Could you check a few things on this model? Use its own coordinates, in mm. A direction names the side the tool comes from. Coordinates: 2 decimals unless noted, no trailing zeros. Loops run counter-clockwise (first coordinate to the right, second up) from the corner with the lowest first, then second, coordinate; pieces in that order, holes last.
1) Imagine slicing it at A-A on x = 14.5. Please give me the cut outline in (y, z).
2) If I drill on line 1 along X through (y, z) = (-6.25, -3.5); line 2 along X through (y, z) = (-6, -5); line 3 along Z through (x, y) = (10.5, -3), over which ranges is the centre line in solid material (lowest first)?
3) For faces 1 (the face through (-6.226, 4.168, 7.179)), 2 (the face through (11.87, -1.08, 4.88)), which set-ups out of +Z, -Z, +X, -X, +Y, -Y let a thin tool reach every point of the face, with its end or its side?
4) Will these pins go through, and if not, where does the flat tip stop? P1, Ø10, axis at x = 13.5, y = 6.5, coming from the +Z side; P2, Ø1.5, axis at y = 5.5, z = -1.5, coming from the +X side; P3, Ø1, axis at x = 4, y = -3, coming from the +Z side.
Autodesk Inventor part; units mm, degrees
ref_plane "Work Plane1" through (1.525, 0, 0) normal (0, 0, 1) x (1, 0, 0)
ref_plane "YZ Plane" through (0, 0, 0) normal (1, 0, 0) x (0, 1, 0)
ref_plane "XZ Plane" through (0, 0, 0) normal (0, 1, 0) x (-1, 0, 0)
sketch "草图1" plane through (0, 0, 0) normal (0, 0, 1) x (1, 0, 0)
  line L0 (0, 7.3) -> (0, 5)
  line L1 (1.5, 5) -> (25, 5)
  line L2 (25, 5) -> (25, 0)
  line L3 (25, 0) -> (-0.6001, 0)
  line L4 (-5.7201, 0) -> (30.12, 0)
  line L5 (-0.6001, 0) -> (-0.6001, 7.3)
  line L6 (-0.6001, 7.3) -> (0, 7.3)
  line L7 (1.5, 5) -> (0.5797, 5)
  line L8 (0.5797, 5) -> (0, 5)
  line L9 (0, -1.46) -> (0, 8.76)
  dimension "d0" = 25
  dimension "d1" = 23.5
  dimension "d2" = 10
  dimension "d9" = 0.6001
  dimension "d10" = 14.6
  dimension "d13" = 0.9203
  dimension "d14" = 10
revolve "轴承体" add sketch "草图1" angle 360 about axis through (25, 0, 0) along (-1, 0, 0)
sketch "草图2" plane through (-0.6001, 0, 0) normal (-1, 0, 0) x (0, 0, 1)
  line L0 (0, 9.2376) -> (8, 4.6188)
  line L1 (8, 4.6188) -> (8, -4.6188)
  line L2 (8, -4.6188) -> (0, -9.2376)
  line L3 (0, -9.2376) -> (-8, -4.6188)
  line L4 (-8, -4.6188) -> (-8, 4.6188)
  line L5 (-8, 4.6188) -> (0, 9.2376)
  point P0 (0, 0)
  point P1 (0, 0)
  dimension "d11" = 16
extrude "头" add sketch "草图2" along normal blind 5.8
sketch "草图4" plane through (0, 0, 0) normal (0, 0, 1) x (1, 0, 0)
  line L0 (-6.4001, 8) -> (-6.4001, 9.2376)
  line L1 (-6.4001, 9.2376) -> (-5.6856, 9.2376)
  line L2 (-5.6856, 9.2376) -> (-6.4001, 8)
  line L3 (-7.5601, 0) -> (0.5599, 0)
  line L4 (-0.6001, 9.2376) -> (-6.4001, 9.2376)
  line L5 (-6.4001, 4.6188) -> (-6.4001, 9.2376)
  dimension "d5" = 30
  dimension "d19" = 16
revolve "倒角1" cut sketch "草图4" angle 360 about axis through (-10, 0, 0) along (1, 0, 0)
thread "螺纹"
chamfer "倒角2" distance 0.9202 distance2 0.9203 1 edges at (25, -5, 0) measured on face at (25, 1.974, 0.2121)
ref_plane "Work Plane1" through (1.525, 0, 0) normal (0, 0, 1) x (1, 0, 0)
equation "\"d11\" = SW"
equation "\"d3\" = KOH - SD"
equation "\"d15\" = GEL"
equation "\"d6\" = -0.5 * SPD + 0.5 * GD"
equation "\"d0\" = NLG"
equation "\"d1\" = GEL"
equation "\"d2\" = GD"
equation "\"d10\" = SD2"
equation "\"d14\" = BDM"
equation "\"d5\" = ANG1"
equation "\"d19\" = SW0"
equation "\"NLG\" = 25"
equation "\"GD\" = NND"
equation "\"BDM\" = NND"
equation "\"KOH\" = 6.4"
equation "\"GEL\" = 23.5"
equation "\"SW\" = 16"
equation "\"SW0\" = SW"
equation "\"SPD\" = NND - 1.2269 * PTC"
equation "\"SD2\" = SDH"
equation "\"SD\" = WFT"
equation "\"ANG1\" = 30deg"
equation "\"GAL\" = 0.61345 * PTC"
equation "\"GUL\" = 0.61345 * PTC"
equation "\"RR\" = 0.4"
equation "\"WFT\" = 0.6"
equation "\"GD1\" = THREADDIA - 1.2269 * PTC"
equation "\"SDH\" = 14.6"
equation "\"TOA\" = 30deg"
equation "\"FAWI\" = 45deg"
equation "\"PTC\" = 1.5"
equation "\"E0\" = 1.155 * SW"
properties part number "螺栓 GB/T 5783 M10 x 25" material "钢，软"
Filled in:
1. outline: circle Ø10 at (0, 0)
2. line 1: x = -6.4 to 0
2. line 2: x = -6.4 to -0.6
2. line 3: z = -4 to 4
3. face 1: +Z, -X, +Y
3. face 2: +X
4. P1: stops at z = 4.77
4. P2: stops at x = 24.13
4. P3: stops at z = 4.33
